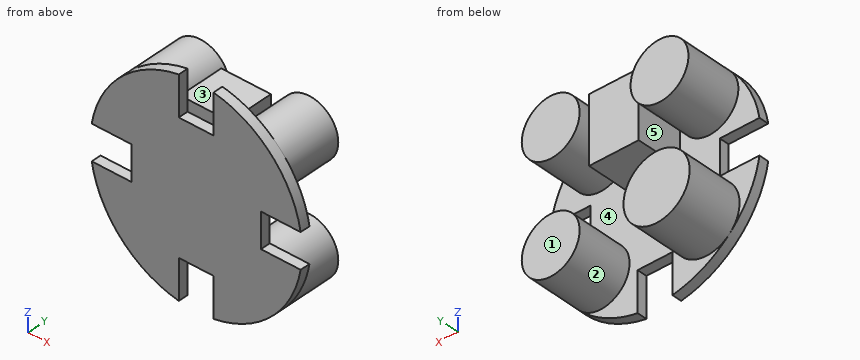
Autodesk Inventor part; units mm, degrees
ref_plane "YZ Plane" through (0, 0, 0) normal (1, 0, 0) x (0, 1, 0)
ref_plane "XZ Plane" through (0, 0, 0) normal (0, 1, 0) x (-1, 0, 0)
ref_plane "XY Plane" through (0, 0, 0) normal (0, 0, 1) x (1, 0, 0)
sketch "Sketch4" plane through (0, 0, 0) normal (0, 1, 0) x (-1, 0, 0)
  circle A0 centre (0, 0) radius 32
  dimension "d48" = 64
extrude "Extrusion1" add sketch "Sketch4" along normal blind 3
sketch "Sketch11" plane through (0, 0, 0) normal (0, -1, 0) x (1, 0, 0)
  point P0 (0, 0)
sketch "Sketch12" plane through (0, 3, 0) normal (0, 1, 0) x (1, 0, 0)
  circle A0 centre (16.4402, -16.4402) radius 8.75
  circle A1 centre (-15.5563, 15.5563) radius 10
  circle A2 centre (-16.4402, -16.4402) radius 8.75
  circle A3 centre (16.4402, 16.4402) radius 8.75
  line L0 (0, 0) -> (-4.7389, -4.7389)
  line L1 (0, 0) -> (6.7018, 0) construction
  line L2 (0, 0) -> (4.7389, -4.7389)
  dimension "d105" = 17.5
  dimension "d106" = 20
  dimension "d107" = 17.5
  dimension "d108" = 17.5
  dimension "d109" = 135
  dimension "d110" = 23.25
  dimension "d111" = 22
  dimension "d112" = 23.25
extrude "Extrusion6" add sketch "Sketch12" along normal blind 17
sketch "Sketch13" plane through (0, 0, 0) normal (0, -1, 0) x (1, 0, 0)
  line L0 (5.25, -39.5664) -> (-5.25, -39.5664)
  line L1 (-5.25, -39.5664) -> (-5.25, -19.5664)
  line L2 (-5.25, -19.5664) -> (5.25, -19.5664)
  line L3 (5.25, -19.5664) -> (5.25, -39.5664)
  line L4 (0, 0) -> (0, -5.0055)
  arc A0 (5.25, -31.5664) -> (-5.25, -31.5664) centre (0, 0) ccw
  arc A1 (-5.25, -31.5664) -> (5.25, -31.5664) centre (0, 0) ccw
  circle A2 centre (0, 0) radius 32
  line L5 (39.5664, 5.25) -> (39.5664, -5.25)
  line L6 (39.5664, -5.25) -> (19.5664, -5.25)
  line L7 (19.5664, -5.25) -> (19.5664, 5.25)
  line L8 (19.5664, 5.25) -> (39.5664, 5.25)
  arc A3 (31.5664, -5.25) -> (31.5664, 5.25) centre (0, 0) ccw
  line L9 (-5.25, 39.5664) -> (5.25, 39.5664)
  line L10 (5.25, 39.5664) -> (5.25, 19.5664)
  line L11 (5.25, 19.5664) -> (-5.25, 19.5664)
  line L12 (-5.25, 19.5664) -> (-5.25, 39.5664)
  arc A4 (5.25, 31.5664) -> (-5.25, 31.5664) centre (0, 0) ccw
  line L13 (-39.5664, -5.25) -> (-39.5664, 5.25)
  line L14 (-39.5664, 5.25) -> (-19.5664, 5.25)
  line L15 (-19.5664, 5.25) -> (-19.5664, -5.25)
  line L16 (-19.5664, -5.25) -> (-39.5664, -5.25)
  arc A5 (-31.5664, 5.25) -> (-31.5664, -5.25) centre (0, 0) ccw
  dimension "d115" = 10.5
  dimension "d116" = 20
  dimension "d117" = 12
  dimension "d118" = 0
  dimension "d121" = 360
extrude "Extrusion7" cut sketch "Sketch13" against normal blind 17 contours A1 L1 L2 L3 | L6 L7 L8 A0 | A0 L14 L15 L16 | A0 L10 L11 L12
sketch "Sketch14" plane through (0, 3, 0) normal (0, 1, 0) x (1, 0, 0)
  line L0 (7.5, -3) -> (-7.5, -3)
  line L1 (-7.5, -3) -> (-7.5, -23)
  line L2 (-7.5, -23) -> (7.5, -23)
  line L3 (7.5, -23) -> (7.5, -3)
  line L4 (0, 0) -> (0, -3.7572)
  dimension "d125" = 15
  dimension "d126" = 20
  dimension "d127" = 3
extrude "Extrusion8" add sketch "Sketch14" along normal blind 14
sketch "Sketch15" plane through (0, 17, 0) normal (0, 1, 0) x (1, 0, 0)
  point P0 (0, 0)
properties part number "Circuit"
Check sheet for the modelled part. Datum: model origin and axes. Units: mm. Face numbers are marked on the shaded views. A direction names the side the tool comes from. Give positions to 0.01 mm unless a question says otherwise; leave off trailing zeros. Loops run counter-clockwise (first coordinate to the right, second up) from the corner with the lowest first, then second, coordinate; pieces in that order, holes last. Notation, with made-up numbers: (48, 61.5) - (70, 61.5) arc R30 cw to (70, 83.5) - close; hole circle Ø6 at (76.5, 6). An arc over 180 degrees is marked (long way). One line per question, with ' | ' between items. Start each with the question number.
1. Cross-section at A-A, the plane x = 26.5. Enter the section's corners in (y, z).
2. Cross-section at D-D, the plane y = 12.25. Enter the section's corners in (x, z), plus the area to 3 significant figures.
3. Cross-section at B-B, the plane z = -26.5. Enter the section's corners in (x, y).
4. Set-up check for the marked faces 1 and 2: record each of +Z, -Z, +X, -X, +Y, -Y from which the full face is reachable in a straight line by a thin tool's end or side.
5. Draft check along Z on the marked faces 3, 4 and 5. Enter one of: released by +Z, released by -Z, zero draft, split by the parting line, or undercut.
6. Material ranges on line 1 along X through (y, z) = (6.5, 13); line 2 along Z through (x, y) = (16.5, 18); line 3 along Y through (x, z) = (-6.5, -5), recorded low to high. Write a range as [from, to].
7. Cross-section at C-C, the plane x = -4. Enter the section's corners in (y, z).
8. Gauge pin test, flat ends, axial feed: pin 1 Ø3.5 at (x, y) = (-25, 1.5) entering from +Z; pin 2 Ø3.5 at (y, z) = (1.5, 25) entering from -X; pin 3 Ø0.9 at (x, y) = (-1.5, 2) entering from +Z; pin 4 Ø3 at (y, z) = (9, 0) entering from -X. Record the tip position at first contact, or that the pin passes through.
Check result:
1) outline: (0, -17.94) - (3, -17.94) - (3, -5.25) - (0, -5.25) - close; (0, 5.25) - (3, 5.25) - (3, 17.94) - (0, 17.94) - close
2) outline: circle Ø20 at (-15.56, -15.56); circle Ø17.5 at (-16.44, 16.44); (-7.5, 3) - (7.5, 3) - (7.5, 23) - (-7.5, 23) - close; circle Ø17.5 at (16.44, -16.44); circle Ø17.5 at (16.44, 16.44) | area: 1,340 mm2
3) outline: (-17.94, 0) - (-5.25, 0) - (-5.25, 3) - (-17.94, 3) - close; (5.25, 0) - (17.94, 0) - (17.94, 3) - (5.25, 3) - close
4) face 1: +Z, -Z, +X, -X, +Y | face 2: +Y
5) face 3: released by +Z | face 4: undercut | face 5: zero draft
6) line 1: x = [-24.49, -8.39], [-7.5, 7.5], [8.39, 24.49] | line 2: z = [-25.19, -7.69], [7.69, 25.19] | line 3: y = [0, 3]
7) outline: (0, -19.57) - (3, -19.57) - (3, 3) - (17, 3) - (17, 23) - (3, 23) - (3, 19.57) - (0, 19.57) - close
8) pin 1: stops at z = 21.99 | pin 2: stops at x = -21.99 | pin 3: stops at z = 19.57 | pin 4: passes through
